The model under review builds one solid part; all positions refer to its coordinate system, in mm. Round coordinates to 2 decimals unless told otherwise and drop trailing zeros. Write each loop counter-clockwise with the first axis right and the second up, starting at its lowest first coordinate (ties: lowest second). Pieces come first, ordered by that corner, then holes. Notation, with made-up numbers: M 32,45 L 40,45 A20 cw 40,67 Z; hole C 32.25,36 d1. An arc over 180 degrees is marked long. One line per item, written item: value. Start each with the question number.
1) For P1, Ø4, axis at x = 10.5, y = -318, coming from the +Z side, flat-tipped, find the tip position at first contact; note if it passes through.
2) Take a section at A-A, the plane y = -410. Write out the cut boundary in (x, z), and give its area (3 significant figures).
3) Wall thickness on probe 1 along Z at (x, y) = (6.5, 116); probe 2 along Z at (x, y) = (1.5, 124.5); probe 3 along X at (y, z) = (21.5, 20.5): over which ranges is each line inside the solid? List them lowest first.
4) Take a section at B-B, the plane x = 7.5. Write out the cut boundary in (y, z), and give its area (3 significant figures).
from build123d import *

# Parameters (mm, degrees)
F0_W     = 1524
F0_H     = 50.8
F1_DEPTH = 19.05
F3_DEPTH = 50.801
F5_DEPTH = 1524.001


# Not quite as in the source:
# - a pattern or mirror of a feature is missing from the dataset's text; its kind, count and spacing are read off the source's solid


with BuildPart() as f1:
    # F0 (on Right) → F1 (new body)
    with BuildSketch(Plane.YZ):
        Rectangle(F0_W, F0_H)
    extrude(amount=F1_DEPTH)

    # F2 (on face) → F3 (cut, through all)
    with BuildSketch(Plane.XY.offset(25.4)):
        Polygon((19.05, 762), (0, 762), (19.05, 742.95), align=None)
    f3 = extrude(amount=-F3_DEPTH, mode=Mode.SUBTRACT)

    # F3_copies: F3 across plane
    add(f3.mirror(Plane(origin=(0, 0, 0), x_dir=(0, 0, -1), z_dir=(0, -1, 0))), mode=Mode.SUBTRACT)

    # F4 (on face) → F5 (cut, through all)
    with BuildSketch(Plane.XZ.offset(762)):
        Polygon((19.05, 25.4), (0, 25.4), (19.05, 6.35), align=None)
    extrude(amount=-F5_DEPTH, mode=Mode.SUBTRACT)


solid = f1.part
Checked values:
1. P1: stops at z = 16.9
2. outline: M 0,-25.4 L 19.05,-25.4 L 19.05,6.35 L 0,25.4 Z
2. area: 786 mm2
3. probe 1: z = -25.4 to 18.9
3. probe 2: z = -25.4 to 23.9
3. probe 3: x = 0 to 4.9
4. outline: M -754.5,-25.4 L 754.5,-25.4 L 754.5,17.9 L -754.5,17.9 Z
4. area: 65,300 mm2
